Geometry: final body of the model. Coordinates: model frame, mm. A direction names the side the tool comes from. Coordinates: 2 decimals unless noted, no trailing zeros. Order: outer loops, then holes, each group sorted by start corner. A loop starts at its lowest first (then second) coordinate and runs counter-clockwise, first axis right, second up. Notation, with made-up numbers: (79.5, 75.25) - (93.5, 75.25) arc R13 ccw to (93.5, 93.25) - close; hole circle Ø10 at (-35.75, 25.5). An arc over 180 degrees is marked (long way). Use a Markdown table: item, result. Add a question column.
```python
from build123d import *

# Parameters (mm, degrees)
SKETCH_1_R      = 2.5
EXTRUDE_1_DEPTH = 200


with BuildPart() as part:
    # 草图1 → 凸台-拉伸1 (new body)
    with BuildSketch(Plane(origin=(0, 0, 0), x_dir=(1, 0, 0), z_dir=(0, 1, 0))):
        with BuildLine():
            Line((-4.415608984, 3.873972711), (-4.415608984, -1.204706946))
            Line((-4.415608984, -1.204706946), (-7.376269156, -4.165367117))
            Line((-7.376269156, -4.165367117), (-9.015608984, -4.165367117))
            Line((-9.015608984, -4.165367117), (-9.015608984, -1.765367117))
            Line((-9.015608984, -1.765367117), (-10.015608984, -1.765367117))
            Line((-10.015608984, -1.765367117), (-10.015608984, -2.265367117))
            Line((-10.015608984, -2.265367117), (-10.815608984, -2.265367117))
            Line((-10.815608984, -2.265367117), (-10.815608984, -7.165367117))
            ThreePointArc((-10.815608984, -7.165367117), (-10.376269156, -8.226027289), (-9.315608984, -8.665367117))
            Line((-9.315608984, -8.665367117), (-4.415608984, -8.665367117))
            Line((-4.415608984, -8.665367117), (-4.415608984, -7.865367117))
            Line((-4.415608984, -7.865367117), (-3.915608984, -7.865367117))
            Line((-3.915608984, -7.865367117), (-3.915608984, -6.865367117))
            Line((-3.915608984, -6.865367117), (-6.315608984, -6.865367117))
            Line((-6.315608984, -6.865367117), (-6.315608984, -5.226027289))
            Line((-6.315608984, -5.226027289), (-3.354948812, -2.265367117))
            Line((-3.354948812, -2.265367117), (1.723730844, -2.265367117))
            Line((1.723730844, -2.265367117), (4.684391016, -5.226027289))
            Line((4.684391016, -5.226027289), (4.684391016, -6.865367117))
            Line((4.684391016, -6.865367117), (2.284391016, -6.865367117))
            Line((2.284391016, -6.865367117), (2.284391016, -7.865367117))
            Line((2.284391016, -7.865367117), (2.784391016, -7.865367117))
            Line((2.784391016, -7.865367117), (2.784391016, -8.665367117))
            Line((2.784391016, -8.665367117), (7.684391016, -8.665367117))
            ThreePointArc((7.684391016, -8.665367117), (8.745051188, -8.226027289), (9.184391016, -7.165367117))
            Line((9.184391016, -7.165367117), (9.184391016, -2.265367117))
            Line((9.184391016, -2.265367117), (8.384391016, -2.265367117))
            Line((8.384391016, -2.265367117), (8.384391016, -1.765367117))
            Line((8.384391016, -1.765367117), (7.384391016, -1.765367117))
            Line((7.384391016, -1.765367117), (7.384391016, -4.165367117))
            Line((7.384391016, -4.165367117), (5.745051188, -4.165367117))
            Line((5.745051188, -4.165367117), (2.784391016, -1.204706946))
            Line((2.784391016, -1.204706946), (2.784391016, 3.873972711))
            Line((2.784391016, 3.873972711), (5.745051188, 6.834632883))
            Line((5.745051188, 6.834632883), (7.384391016, 6.834632883))
            Line((7.384391016, 6.834632883), (7.384391016, 4.434632883))
            Line((7.384391016, 4.434632883), (8.384391016, 4.434632883))
            Line((8.384391016, 4.434632883), (8.384391016, 4.934632883))
            Line((8.384391016, 4.934632883), (9.184391016, 4.934632883))
            Line((9.184391016, 4.934632883), (9.184391016, 9.834632883))
            ThreePointArc((9.184391016, 9.834632883), (8.745051188, 10.895293054), (7.684391016, 11.334632883))
            Line((7.684391016, 11.334632883), (2.784391016, 11.334632883))
            Line((2.784391016, 11.334632883), (2.784391016, 10.534632883))
            Line((2.784391016, 10.534632883), (2.284391016, 10.534632883))
            Line((2.284391016, 10.534632883), (2.284391016, 9.534632883))
            Line((2.284391016, 9.534632883), (4.684391016, 9.534632883))
            Line((4.684391016, 9.534632883), (4.684391016, 7.895293054))
            Line((4.684391016, 7.895293054), (1.723730844, 4.934632883))
            Line((1.723730844, 4.934632883), (-3.354948812, 4.934632883))
            Line((-3.354948812, 4.934632883), (-6.315608984, 7.895293054))
            Line((-6.315608984, 7.895293054), (-6.315608984, 9.534632883))
            Line((-6.315608984, 9.534632883), (-3.915608984, 9.534632883))
            Line((-3.915608984, 9.534632883), (-3.915608984, 10.534632883))
            Line((-3.915608984, 10.534632883), (-4.415608984, 10.534632883))
            Line((-4.415608984, 10.534632883), (-4.415608984, 11.334632883))
            Line((-4.415608984, 11.334632883), (-9.315608984, 11.334632883))
            ThreePointArc((-9.315608984, 11.334632883), (-10.376269156, 10.895293054), (-10.815608984, 9.834632883))
            Line((-10.815608984, 9.834632883), (-10.815608984, 4.934632883))
            Line((-10.815608984, 4.934632883), (-10.015608984, 4.934632883))
            Line((-10.015608984, 4.934632883), (-10.015608984, 4.434632883))
            Line((-10.015608984, 4.434632883), (-9.015608984, 4.434632883))
            Line((-9.015608984, 4.434632883), (-9.015608984, 6.834632883))
            Line((-9.015608984, 6.834632883), (-7.376269156, 6.834632883))
            Line((-7.376269156, 6.834632883), (-4.415608984, 3.873972711))
        make_face()
        with Locations(Location((-0.815608984, 1.334632883, 0), (0, 0, 270))):
            Circle(SKETCH_1_R, mode=Mode.SUBTRACT)
    extrude(amount=EXTRUDE_1_DEPTH)


solid = part.part
```
1) Access query for faces 5 (the flat face through (-1, 99, 2.265)), 6 (the flat face through (2.784, 99, -1)), 7 (the flat face through (-1, 99, -4.935)). Directions: +Z, -Z, +X, -X, +Y, -Y. A direction counts if a zero-diameter tool reaches every point of the face in a straight line with its end or side. Return the directions, or none.
2) First-contact query: pin 1 (5.5 mm diameter, centred on y = 65, z = -2, fed in from -X); pin 2 (1.5 mm diameter, centred on x = 0, y = 137, fed in from -Z). Flat tips, straight axial feed; report the tip coordinate or a pass-through.
3) Line query: line 1 (X direction, y = 189.5, z = -1.25); line 2 (X direction, y = 106.5, z = 5.75); line 3 (Z direction, x = 3.25, y = 165.5). Output: solid intervals per line, ascending. Write a range as from..to.
4) Section query A-A (z = -2). Return the cut outline in (x, y), and give its area (3 significant figures).
5) Draft query along X for faces 1 (the flat face through (-3, 0, -4)), 2 (the flat face through (-4.416, 99, -1)), 3 (the flat face through (9.184, 99, 5)), 4 (the cylindrical face through (-0.706, 98.6, -3.832)). Return one class per face: released by +X, released by -X, zero draft, split by the parting line, or undercut.
From the geometry:
| question | item | result |
|---|---|---|
| 1 | face 5 | +Z, +Y, -Y |
| 1 | face 6 | +X, +Y, -Y |
| 1 | face 7 | -Z, +Y, -Y |
| 2 | pin 1 | stops at x = -10.02 |
| 2 | pin 2 | stops at z = -4.93 |
| 3 | line 1 | x = -4.42..-3.31, 1.68..2.78 |
| 3 | line 2 | x = -10.82..-6.32, 4.68..9.18 |
| 3 | line 3 | z = -11.33..-9.53, -6.46..-4.34, 1.67..3.79, 6.87..8.67 |
| 4 | outline | (-4.42, 0) - (-3.23, 0) - (-3.23, 200) - (-4.42, 200) - close; (1.59, 0) - (2.78, 0) - (2.78, 200) - (1.59, 200) - close |
| 4 | area | 476 mm^2 |
| 5 | face 1 | zero draft |
| 5 | face 2 | released by -X |
| 5 | face 3 | released by +X |
| 5 | face 4 | undercut |
